Geometry: final body of the model. Coordinates: model frame, mm. Give positions to 0.01 mm unless a question says otherwise; leave off trailing zeros. Write each loop counter-clockwise with the first axis right and the second up, starting at its lowest first coordinate (ties: lowest second). Pieces come first, ordered by that corner, then holes. Notation, with made-up numbers: (41, -8) -> (48, -8) arc R16 cw to (48, 22) -> close; hole circle Ø9 at (-3.5, 6). An arc over 180 degrees is marked (long way). Use CSV: the item, a comma, the result in double quotes. Start each with the question number.
1) Contact query for flat-ended pins moving along their axis: P1, Ø4, axis at x = 15.5, z = -17.5, coming from the -Y side; P2, Ø1.3, axis at x = -26.5, y = 4, coming from the +Z side; P3, Ø1.5, axis at y = 3.5, z = -16.5, coming from the -X side; P4, Ø0.5, axis at x = -1, y = 2, coming from the -Z side. Output: stop coordinate, or through.
2) Material intervals for line 1 (X direction, y = 4.75, z = 0); line 2 (Z direction, x = 0, y = 4.25); line 3 (Z direction, x = -19, y = 4.75), sorted ascending. Write a range as [from, to].
3) Section A-A (z = 0). Output: boundary loops of the cut face in (x, y), plus the area to 3 significant figures.
4) Section B-B (x = 8). Output: boundary loops of the cut face in (y, z).
```python
from build123d import *

# Parameters (mm, degrees)
SKETCH1_R           = 25.4
SKETCH1_W           = 1.814083278
SKETCH1_H           = 1.595577256
SKETCH1_W_2         = 1.595577256
SKETCH1_H_2         = 1.814083278
BOSS_EXTRUDE1_DEPTH = 6.35


with BuildPart() as part:
    # Sketch1 → Boss-Extrude1 (new body)
    # profile 1 of 33: a face of its own
    with BuildSketch(Plane(origin=(0, 0, 0), x_dir=(1, 0, 0), z_dir=(0, 1, 0))):
        Circle(SKETCH1_R)
        with BuildLine():
            Line((-0.62166438, 6.319496293), (-0.62166438, 5.475030088))
            Line((-0.62166438, 5.475030088), (0.308287629, 5.475030088))
            Line((0.308287629, 5.475030088), (0.308287629, 6.342512021))
            ThreePointArc((0.308287629, 6.342512021), (0.1571104, -6.348056106), (-0.62166438, 6.319496293))
        make_face(mode=Mode.SUBTRACT)
    # profile 2 of 33: a face of its own
    with BuildSketch(Plane(origin=(0, 0, 0), x_dir=(1, 0, 0), z_dir=(0, 1, 0))):
        Polygon((4.655372194, 26.590682963), (6.434598369, 26.236772872), (6.123316689, 24.671854186), (4.344090513, 25.025764276), align=None)
    # profile 3 of 33: a face of its own
    with BuildSketch(Plane(origin=(0, 0, 0), x_dir=(1, 0, 0), z_dir=(0, 1, 0))):
        with Locations((0.285377259, 26.190179878)):
            Rectangle(SKETCH1_W, SKETCH1_H)
    # profile 4 of 33: a face of its own
    with BuildSketch(Plane(origin=(0, 0, 0), x_dir=(1, 0, 0), z_dir=(0, 1, 0))):
        Polygon((9.753505424, 25.171532385), (11.429499834, 24.47731277), (10.818898853, 23.003191601), (9.142904443, 23.697411216), align=None)
    # profile 5 of 33: a face of its own
    with BuildSketch(Plane(origin=(0, 0, 0), x_dir=(1, 0, 0), z_dir=(0, 1, 0))):
        Polygon((14.476816911, 22.785053935), (15.98517203, 21.777203266), (15.098716802, 20.450529263), (13.590361683, 21.458379932), align=None)
    # profile 6 of 33: a face of its own
    with BuildSketch(Plane(origin=(0, 0, 0), x_dir=(1, 0, 0), z_dir=(0, 1, 0))):
        Polygon((18.643792443, 19.52295864), (19.92654303, 18.240208053), (18.798299532, 17.111964555), (17.515548945, 18.394715142), align=None)
    # profile 7 of 33: a face of its own
    with BuildSketch(Plane(origin=(0, 0, 0), x_dir=(1, 0, 0), z_dir=(0, 1, 0))):
        Polygon((22.094297486, 15.510606992), (23.102148155, 14.002251873), (21.775474153, 13.115796645), (20.767623484, 14.624151764), align=None)
    # profile 8 of 33: a face of its own
    with BuildSketch(Plane(origin=(0, 0, 0), x_dir=(1, 0, 0), z_dir=(0, 1, 0))):
        Polygon((24.695731068, 10.902191417), (25.389950683, 9.226197007), (23.915829514, 8.615596026), (23.221609899, 10.291590436), align=None)
    # profile 9 of 33: a face of its own
    with BuildSketch(Plane(origin=(0, 0, 0), x_dir=(1, 0, 0), z_dir=(0, 1, 0))):
        Polygon((26.348121555, 5.874810739), (26.702031645, 4.095584564), (25.137112959, 3.784302883), (24.783202868, 5.563529059), align=None)
    # profile 10 of 33: a face of its own
    with BuildSketch(Plane(origin=(0, 0, 0), x_dir=(1, 0, 0), z_dir=(0, 1, 0))):
        with Locations((26.190179878, -0.285377259)):
            Rectangle(SKETCH1_W_2, SKETCH1_H_2)
    # profile 11 of 33: a face of its own
    with BuildSketch(Plane(origin=(0, 0, 0), x_dir=(1, 0, 0), z_dir=(0, 1, 0))):
        Polygon((26.590682963, -4.655372194), (26.236772872, -6.434598369), (24.671854186, -6.123316689), (25.025764276, -4.344090513), align=None)
    # profile 12 of 33: a face of its own
    with BuildSketch(Plane(origin=(0, 0, 0), x_dir=(1, 0, 0), z_dir=(0, 1, 0))):
        Polygon((25.171532385, -9.753505424), (24.47731277, -11.429499834), (23.003191601, -10.818898853), (23.697411216, -9.142904443), align=None)
    # profile 13 of 33: a face of its own
    with BuildSketch(Plane(origin=(0, 0, 0), x_dir=(1, 0, 0), z_dir=(0, 1, 0))):
        Polygon((22.785053935, -14.476816911), (21.777203266, -15.98517203), (20.450529263, -15.098716802), (21.458379932, -13.590361683), align=None)
    # profile 14 of 33: a face of its own
    with BuildSketch(Plane(origin=(0, 0, 0), x_dir=(1, 0, 0), z_dir=(0, 1, 0))):
        Polygon((19.52295864, -18.643792443), (18.240208053, -19.92654303), (17.111964555, -18.798299532), (18.394715142, -17.515548945), align=None)
    # profile 15 of 33: a face of its own
    with BuildSketch(Plane(origin=(0, 0, 0), x_dir=(1, 0, 0), z_dir=(0, 1, 0))):
        Polygon((15.510606992, -22.094297486), (14.002251873, -23.102148155), (13.115796645, -21.775474153), (14.624151764, -20.767623484), align=None)
    # profile 16 of 33: a face of its own
    with BuildSketch(Plane(origin=(0, 0, 0), x_dir=(1, 0, 0), z_dir=(0, 1, 0))):
        Polygon((10.902191417, -24.695731068), (9.226197007, -25.389950683), (8.615596026, -23.915829514), (10.291590436, -23.221609899), align=None)
    # profile 17 of 33: a face of its own
    with BuildSketch(Plane(origin=(0, 0, 0), x_dir=(1, 0, 0), z_dir=(0, 1, 0))):
        Polygon((5.874810739, -26.348121555), (4.095584564, -26.702031645), (3.784302883, -25.137112959), (5.563529059, -24.783202868), align=None)
    # profile 18 of 33: a face of its own
    with BuildSketch(Plane(origin=(0, 0, 0), x_dir=(1, 0, 0), z_dir=(0, 1, 0))):
        with Locations((-0.285377259, -26.190179878)):
            Rectangle(SKETCH1_W, SKETCH1_H)
    # profile 19 of 33: a face of its own
    with BuildSketch(Plane(origin=(0, 0, 0), x_dir=(1, 0, 0), z_dir=(0, 1, 0))):
        Polygon((-4.655372194, -26.590682963), (-6.434598369, -26.236772872), (-6.123316689, -24.671854186), (-4.344090513, -25.025764276), align=None)
    # profile 20 of 33: a face of its own
    with BuildSketch(Plane(origin=(0, 0, 0), x_dir=(1, 0, 0), z_dir=(0, 1, 0))):
        Polygon((-9.753505424, -25.171532385), (-11.429499834, -24.47731277), (-10.818898853, -23.003191601), (-9.142904443, -23.697411216), align=None)
    # profile 21 of 33: a face of its own
    with BuildSketch(Plane(origin=(0, 0, 0), x_dir=(1, 0, 0), z_dir=(0, 1, 0))):
        Polygon((-14.476816911, -22.785053935), (-15.98517203, -21.777203266), (-15.098716802, -20.450529263), (-13.590361683, -21.458379932), align=None)
    # profile 22 of 33: a face of its own
    with BuildSketch(Plane(origin=(0, 0, 0), x_dir=(1, 0, 0), z_dir=(0, 1, 0))):
        Polygon((-18.643792443, -19.52295864), (-19.92654303, -18.240208053), (-18.798299532, -17.111964555), (-17.515548945, -18.394715142), align=None)
    # profile 23 of 33: a face of its own
    with BuildSketch(Plane(origin=(0, 0, 0), x_dir=(1, 0, 0), z_dir=(0, 1, 0))):
        Polygon((-22.094297486, -15.510606992), (-23.102148155, -14.002251873), (-21.775474153, -13.115796645), (-20.767623484, -14.624151764), align=None)
    # profile 24 of 33: a face of its own
    with BuildSketch(Plane(origin=(0, 0, 0), x_dir=(1, 0, 0), z_dir=(0, 1, 0))):
        Polygon((-24.695731068, -10.902191417), (-25.389950683, -9.226197007), (-23.915829514, -8.615596026), (-23.221609899, -10.291590436), align=None)
    # profile 25 of 33: a face of its own
    with BuildSketch(Plane(origin=(0, 0, 0), x_dir=(1, 0, 0), z_dir=(0, 1, 0))):
        Polygon((-26.348121555, -5.874810739), (-26.702031645, -4.095584564), (-25.137112959, -3.784302883), (-24.783202868, -5.563529059), align=None)
    # profile 26 of 33: a face of its own
    with BuildSketch(Plane(origin=(0, 0, 0), x_dir=(1, 0, 0), z_dir=(0, 1, 0))):
        with Locations((-26.190179878, 0.285377259)):
            Rectangle(SKETCH1_W_2, SKETCH1_H_2)
    # profile 27 of 33: a face of its own
    with BuildSketch(Plane(origin=(0, 0, 0), x_dir=(1, 0, 0), z_dir=(0, 1, 0))):
        Polygon((-26.590682963, 4.655372194), (-26.236772872, 6.434598369), (-24.671854186, 6.123316689), (-25.025764276, 4.344090513), align=None)
    # profile 28 of 33: a face of its own
    with BuildSketch(Plane(origin=(0, 0, 0), x_dir=(1, 0, 0), z_dir=(0, 1, 0))):
        Polygon((-25.171532385, 9.753505424), (-24.47731277, 11.429499834), (-23.003191601, 10.818898853), (-23.697411216, 9.142904443), align=None)
    # profile 29 of 33: a face of its own
    with BuildSketch(Plane(origin=(0, 0, 0), x_dir=(1, 0, 0), z_dir=(0, 1, 0))):
        Polygon((-22.785053935, 14.476816911), (-21.777203266, 15.98517203), (-20.450529263, 15.098716802), (-21.458379932, 13.590361683), align=None)
    # profile 30 of 33: a face of its own
    with BuildSketch(Plane(origin=(0, 0, 0), x_dir=(1, 0, 0), z_dir=(0, 1, 0))):
        Polygon((-19.52295864, 18.643792443), (-18.240208053, 19.92654303), (-17.111964555, 18.798299532), (-18.394715142, 17.515548945), align=None)
    # profile 31 of 33: a face of its own
    with BuildSketch(Plane(origin=(0, 0, 0), x_dir=(1, 0, 0), z_dir=(0, 1, 0))):
        Polygon((-15.510606992, 22.094297486), (-14.002251873, 23.102148155), (-13.115796645, 21.775474153), (-14.624151764, 20.767623484), align=None)
    # profile 32 of 33: a face of its own
    with BuildSketch(Plane(origin=(0, 0, 0), x_dir=(1, 0, 0), z_dir=(0, 1, 0))):
        Polygon((-10.902191417, 24.695731068), (-9.226197007, 25.389950683), (-8.615596026, 23.915829514), (-10.291590436, 23.221609899), align=None)
    # profile 33 of 33: a face of its own
    with BuildSketch(Plane(origin=(0, 0, 0), x_dir=(1, 0, 0), z_dir=(0, 1, 0))):
        Polygon((-5.874810739, 26.348121555), (-4.095584564, 26.702031645), (-3.784302883, 25.137112959), (-5.563529059, 24.783202868), align=None)
    extrude(amount=BOSS_EXTRUDE1_DEPTH)


solid = part.part
```
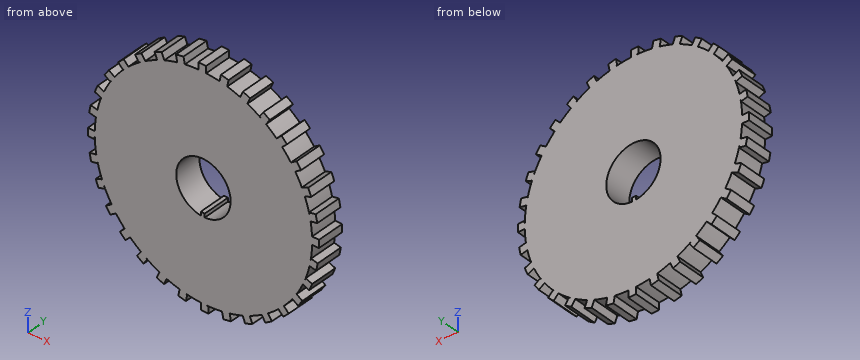
Answers follow:
1,P1,"stops at y = 0"
1,P2,"stops at z = 5.87"
1,P3,"stops at x = -21.93"
1,P4,"stops at z = -25.39"
2,line 1,"x = [-26.99, -6.35], [6.35, 26.99]"
2,line 2,"z = [-26.99, -5.48], [6.35, 26.99]"
2,line 3,"z = [-19.17, -18.12], [-16.86, 16.86], [17.31, 19.17]"
3,outline,"(-26.99, 0) -> (-6.35, 0) -> (-6.35, 6.35) -> (-26.99, 6.35) -> close; (6.35, 0) -> (26.99, 0) -> (26.99, 6.35) -> (6.35, 6.35) -> close"
3,area,"262 mm^2"
4,outline,"(0, -24.11) -> (6.35, -24.11) -> (6.35, 24.11) -> (0, 24.11) -> close"
